Geometry: final body of the model. Coordinates: model frame, mm. Face numbers are marked on the shaded views. A direction names the side the tool comes from. Coordinates: 2 decimals unless noted, no trailing zeros. Write each loop counter-clockwise with the first axis right and the second up, starting at its lowest first coordinate (ties: lowest second). Pieces come first, ordered by that corner, then holes. Notation, with made-up numbers: (-33.75, 48.5) -> (-19.75, 48.5) arc R25 ccw to (-19.75, 82.5) -> close; hole circle Ø2 at (43.5, 59). An arc over 180 degrees is marked (long way). One line per item, written item: value.
```python
from build123d import *

# Parameters (mm, degrees)
SKETCH1_R           = 15
SKETCH1_R_2         = 1
BOSS_EXTRUDE1_DEPTH = 5
SKETCH2_R           = 6
BOSS_EXTRUDE2_DEPTH = 1
SKETCH3_R           = 3
CUT_EXTRUDE1_DEPTH  = 5
SKETCH4_R           = 1.5
CUT_EXTRUDE2_DEPTH  = 5


with BuildPart() as part:
    # Sketch1 → Boss-Extrude1 (new body)
    with BuildSketch(Plane(origin=(0, 0, 0), x_dir=(1, 0, 0), z_dir=(0, 1, 0))):
        with Locations(Location((0, 0, 0), (0, 0, 270))):
            Circle(SKETCH1_R)
        with Locations(Location((0, 12, 0), (0, 0, 270))):
            Circle(SKETCH1_R_2, mode=Mode.SUBTRACT)
        with Locations(Location((8.485281374, 8.485281374, 0), (0, 0, 270))):
            Circle(SKETCH1_R_2, mode=Mode.SUBTRACT)
        with Locations(Location((12, 0, 0), (0, 0, 270))):
            Circle(SKETCH1_R_2, mode=Mode.SUBTRACT)
        with Locations(Location((8.485281374, -8.485281374, 0), (0, 0, 270))):
            Circle(SKETCH1_R_2, mode=Mode.SUBTRACT)
        with Locations(Location((0, -12, 0), (0, 0, 270))):
            Circle(SKETCH1_R_2, mode=Mode.SUBTRACT)
        with Locations(Location((-8.485281374, -8.485281374, 0), (0, 0, 270))):
            Circle(SKETCH1_R_2, mode=Mode.SUBTRACT)
        with Locations(Location((-12, 0, 0), (0, 0, 270))):
            Circle(SKETCH1_R_2, mode=Mode.SUBTRACT)
        with Locations(Location((-8.485281374, 8.485281374, 0), (0, 0, 270))):
            Circle(SKETCH1_R_2, mode=Mode.SUBTRACT)
    extrude(amount=BOSS_EXTRUDE1_DEPTH)

    # Sketch2 → Boss-Extrude2 (add)
    with BuildSketch(Plane(origin=(0, 5, 0), x_dir=(1, 0, 0), z_dir=(0, 1, 0))):
        with Locations(Location((0, 0, 0), (0, 0, 270))):
            Circle(SKETCH2_R)
    extrude(amount=BOSS_EXTRUDE2_DEPTH)

    # Sketch3 → Cut-Extrude1 (cut)
    with BuildSketch(Plane.XZ):
        with Locations(Location((0, 0, 0), (0, 0, 270))):
            Circle(SKETCH3_R)
    extrude(amount=-CUT_EXTRUDE1_DEPTH, mode=Mode.SUBTRACT)

    # Sketch4 → Cut-Extrude2 (cut)
    with BuildSketch(Plane(origin=(0, 6, 0), x_dir=(1, 0, 0), z_dir=(0, 1, 0))):
        with Locations(Location((0, 0, 0), (0, 0, 270))):
            Circle(SKETCH4_R)
    extrude(amount=-CUT_EXTRUDE2_DEPTH, mode=Mode.SUBTRACT)


solid = part.part
```
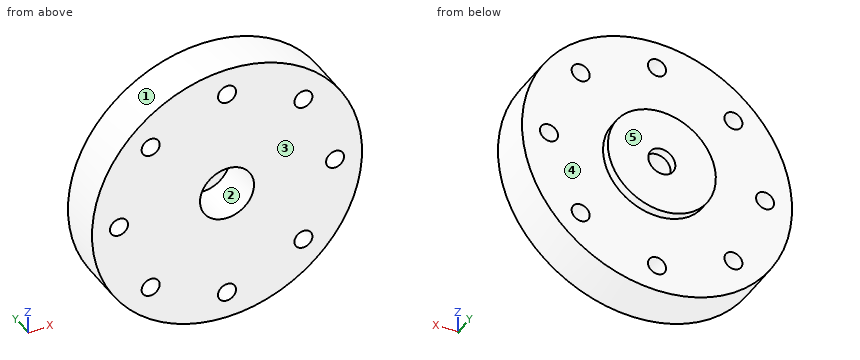
(1) Line query: line 1 (X direction, y = 4, z = 0); line 2 (X direction, y = 0.85, z = -9); line 3 (Y direction, x = 9.5, z = -7.75). Output: solid intervals per line, ascending. Write a range as [from, to].
Responses:
line 1: x = [-15, -13], [-11, -3], [3, 11], [13, 15]
line 2: x = [-12, -9.34], [-7.63, 7.63], [9.34, 12]
line 3: y = [0, 5]
(2) Section B-B (x = 0). Return the cut outline in (y, z).
Responses:
outline: (0, -15) -> (5, -15) -> (5, -13) -> (0, -13) -> close; (0, -11) -> (5, -11) -> (5, -6) -> (6, -6) -> (6, -1.5) -> (5, -1.5) -> (5, -3) -> (0, -3) -> close; (0, 3) -> (5, 3) -> (5, 1.5) -> (6, 1.5) -> (6, 6) -> (5, 6) -> (5, 11) -> (0, 11) -> close; (0, 13) -> (5, 13) -> (5, 15) -> (0, 15) -> close
(3) Section C-C (z = 0). Return the cut outline in (x, y), then the cut area to 3 significant figures.
Responses:
outline: (-15, 0) -> (-13, 0) -> (-13, 5) -> (-15, 5) -> close; (-11, 0) -> (-3, 0) -> (-3, 5) -> (-1.5, 5) -> (-1.5, 6) -> (-6, 6) -> (-6, 5) -> (-11, 5) -> close; (1.5, 5) -> (3, 5) -> (3, 0) -> (11, 0) -> (11, 5) -> (6, 5) -> (6, 6) -> (1.5, 6) -> close; (13, 0) -> (15, 0) -> (15, 5) -> (13, 5) -> close
area: 109 mm2
(4) First-contact query: pin 1 (1 mm diameter, centred on x = -3.5, y = 0.5, fed in from +Z); pin 2 (3 mm diameter, centred on x = 0, z = 12, fed in from +Y); pin 3 (3 mm diameter, centred on y = 1.5, z = 2, fed in from -X). Flat tips, straight axial feed; report the tip coordinate or a pass-through.
Responses:
pin 1: stops at z = 14.7
pin 2: stops at y = 5
pin 3: stops at x = -14.99
(5) Pull-direction query (Z, two-part tool) for the marked faces 1, 2 and 3; classes: released by +Z, released by -Z, zero draft, split by the parting line, or undercut.
Responses:
face 1: split by the parting line
face 2: undercut
face 3: zero draft
(6) Reachability of the marked faces 4 and 5 from +Z, -Z, +X, -X, +Y, -Y: full face, straight path, thin tool, end or side. Return the list, or none.
Responses:
face 4: +Y
face 5: +Z, -Z, +X, -X, +Y
(7) Section D-D (y = 2.05). State how many separate pieces and enclosed holes the cut face has, then the cut area to 3 significant figures.
Responses:
separate pieces: 1
enclosed holes: 9
area: 653 mm2
(8) Section A-A (x = 12). Return the cut outline in (y, z).
Responses:
outline: (0, -9) -> (5, -9) -> (5, -1) -> (0, -1) -> close; (0, 1) -> (5, 1) -> (5, 9) -> (0, 9) -> close
